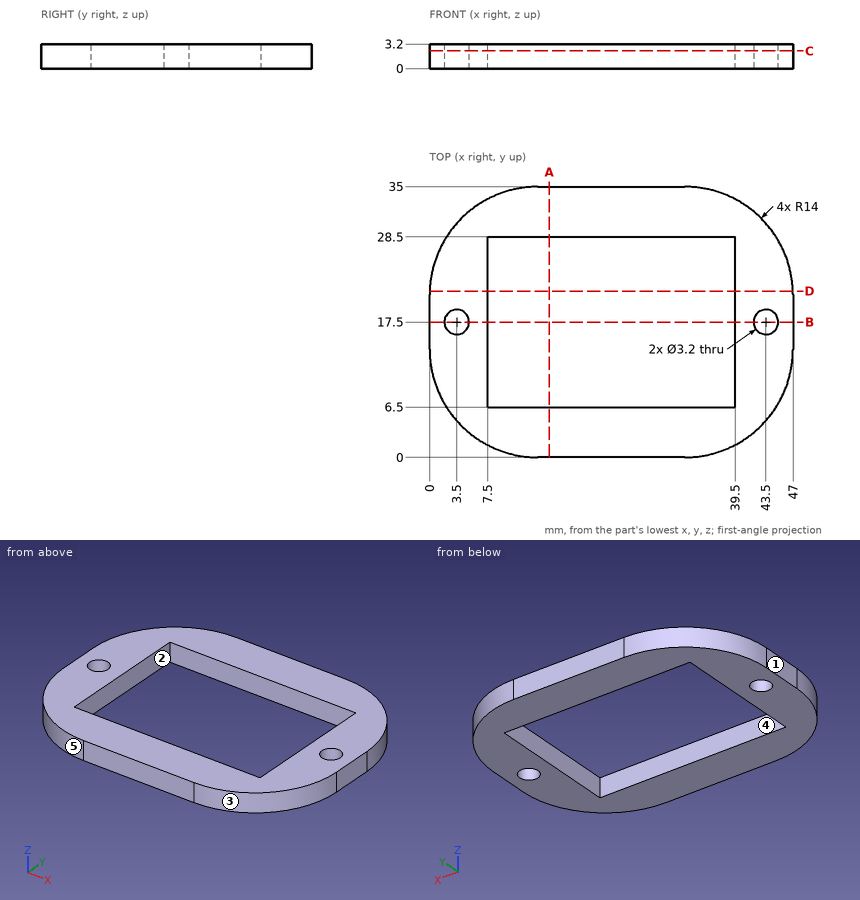
Design review of the part shown in the three views and the two pictorial views. Dimensions are in mm from the part's minimum x, y and z. A direction names the side the tool comes from. Round coordinates to 2 decimals unless told otherwise and drop trailing zeros. Write each loop counter-clockwise with the first axis right and the second up, starting at its lowest first coordinate (ties: lowest second). Pieces come first, ordered by that corner, then holes.
1) Insertion check: pin 1 Ø1.5 at (y, z) = (23, 0.5) entering from -X. The pin has a flat end and moves straight along its axis. Give the tip position at first contact, or say it passes through.
Answer below:
pin 1: stops at x = 0.06
2) Take a section at D-D on y = 21.5. Give the boundary of the cut face in (x, z), then the cut area to 3 significant figures.
Answer below:
outline: (0.01, 0) - (7.5, 0) - (7.5, 3.2) - (0.01, 3.2) - close; (39.5, 0) - (46.99, 0) - (46.99, 3.2) - (39.5, 3.2) - close
area: 47.9 mm2
3) Machinability: for the marked faces 4 and 5, which of the approach directions +Z, -Z, +X, -X, +Y, -Y give a long, thin tool a straight path to every point of the face, cutting with its end or side? Answer none if there is none.
Answer below:
face 4: +Z, -Z
face 5: +Z, -Z, -X, -Y
4) For line 1 along Y through (x, z) = (22, 2); line 2 along X through (y, z) = (21.5, 0.25); line 3 along X through (y, z) = (17, 1.7), list the stretches that pass through material, from the lowest coordinate up.
Answer below:
line 1: y = 0 to 6.5, 28.5 to 35
line 2: x = 0.01 to 7.5, 39.5 to 46.99
line 3: x = 0 to 1.98, 5.02 to 7.5, 39.5 to 41.98, 45.02 to 47
5) Take a section at B-B on y = 17.5. Give the boundary of the cut face in (x, z).
Answer below:
outline: (0, 0) - (1.9, 0) - (1.9, 3.2) - (0, 3.2) - close; (5.1, 0) - (7.5, 0) - (7.5, 3.2) - (5.1, 3.2) - close; (39.5, 0) - (41.9, 0) - (41.9, 3.2) - (39.5, 3.2) - close; (45.1, 0) - (47, 0) - (47, 3.2) - (45.1, 3.2) - close
6) Take a section at C-C on z = 2.3. Give the boundary of the cut face in (x, y).
Answer below:
outline: (0, 14) arc R14 ccw to (14, 0) - (33, 0) arc R14 ccw to (47, 14) - (47, 21) arc R14 ccw to (33, 35) - (14, 35) arc R14 ccw to (0, 21) - close; hole circle Ø3.2 at (3.5, 17.5); hole (7.5, 6.5) - (39.5, 6.5) - (39.5, 28.5) - (7.5, 28.5) - close; hole circle Ø3.2 at (43.5, 17.5)
7) Mouldability with a two-part tool opening along Y and no side actions: class the marked faces 1, 2 and 3 as +Y half, -Y half, draft (parallel to the pull), parting line (faces both ways), or undercut.
Answer below:
face 1: draft
face 2: undercut
face 3: -Y half
8) Take a section at A-A on x = 15.5. Give the boundary of the cut face in (y, z).
Answer below:
outline: (0, 0) - (6.5, 0) - (6.5, 3.2) - (0, 3.2) - close; (28.5, 0) - (35, 0) - (35, 3.2) - (28.5, 3.2) - close
